from build123d import *

# Parameters (mm, degrees)
F1_DEPTH = 6
F2_R     = 3
F3_R     = 2.5
F4_DEPTH = 10
F5_R     = 2.5
F6_DEPTH = 10


with BuildPart() as f1:
    # F0 (on Right) → F1 (new body, symmetric)
    with BuildSketch(Plane.YZ):
        Polygon((0, 150), (-100, 0), (0, 0), align=None)
        Polygon((-10, 10), (-81.314829, 10), (-10, 116.972244), align=None, mode=Mode.SUBTRACT)
    extrude(amount=F1_DEPTH, both=True)

    # F2
    f2_edges = [f1.edges().sort_by_distance(p)[0] for p in [
        (0, -100, 0),
        (0, 0, 150),
        (0, -10, 116.972244),
        (0, -10, 10),
        (0, -81.314829, 10),
    ]]
    fillet(f2_edges, radius=F2_R)

    # F3 (on face) → F4 (cut, through all)
    with BuildSketch(Plane(origin=(0, 0, 0), x_dir=(-1, 0, 0), z_dir=(0, 1, 0))):
        with Locations((0, 90)):
            Circle(F3_R)
        with Locations((0, 25)):
            Circle(F3_R)
    extrude(amount=-F4_DEPTH, mode=Mode.SUBTRACT)

    # F5 (on face) → F6 (cut, through all)
    with BuildSketch(Plane(origin=(0, 0, 0), x_dir=(1, 0, 0), z_dir=(0, 0, -1))):
        with Locations((0, 25)):
            Circle(F5_R)
        with Locations((0, 65)):
            Circle(F5_R)
    extrude(amount=-F6_DEPTH, mode=Mode.SUBTRACT)


solid = f1.part
Here's how the part is built. I have some questions about the finished solid (model axes, mm). A direction names the side the tool comes from. Coordinates: 2 decimals unless noted, no trailing zeros. Loops run counter-clockwise (first coordinate to the right, second up) from the corner with the lowest first, then second, coordinate; pieces in that order, holes last. Notation, with made-up numbers: (4.25, 36) -> (43.25, 36) arc R22 cw to (43.25, 69) -> close; hole circle Ø9 at (17, 39.25). An arc over 180 degrees is marked (long way). Use one line per item in the form item = value. Start each with the question number.
(1) If we section it at D-D (y = -71): Please give me the cut outline in (x, z).
(2) Will these pins go through, and if not, where does the flat tip stop? pin 1 (3.5 mm diameter, centred on x = 1.5, z = 44.5, fed in from -Y); pin 2 (6 mm diameter, centred on x = 0.5, y = -60, fed in from +Z); pin 3 (3 mm diameter, centred on x = 0, y = -25, fed in from +Z).
(3) If we section it at C-C (x = 1): Please give me the cut outline in (y, z), then the cut area to 3 significant figures.
(4) Please list where these lines run through material, in increasing order: line 1 along Y through (x, z) = (0, 2.75); line 2 along Z through (x, y) = (0, -7.25) (3 decimals); line 3 along Y through (x, z) = (0, 6.75).
(5) We'd pull the mould along Z, two halves only. Please class faces 1 (the face through (-0.33, -27.48, 4.93)), 2 (the face through (0.084, -50.554, 74.17)), 3 (the face through (0.08, -10.9, 10.86)): pulls with the +Z half, pulls with the -Z half, needs draft (parallel to the pull), parting line crosses it, or undercut.
(6) If we section it at B-B (z = 71.5): Please give me the cut outline in (x, y), then the cut area to 3 significant figures.
(7) If we section it at A-A (y = -8.5): Please give me the cut outline in (x, z), then the cut area to 3 significant figures.
(8) On a 3-axis mill with a long thin cutter (end or side, diameter ignored), from which of +Z, -Z, +X, -X, +Y, -Y can I reach the whole of each face in a straight line? I mean faces 4 (the face through (0.33, -4.93, 27.48)), 5 (the face through (0.08, -47.29, 61.04)), 6 (the face through (-0.33, -67.48, 4.93)). Say none if no direction works.
Verdict:
q1.outline = (-6, 0) -> (6, 0) -> (6, 10) -> (-6, 10) -> close; (-6, 25.47) -> (6, 25.47) -> (6, 43.5) -> (-6, 43.5) -> close
q2.pin_1 = -71.5
q2.pin_2 = 64.5
q2.pin_3 = 114.75
q3.outline = (-96.89, 4.66) arc R3 ccw to (-94.39, 0) -> (-67.29, 0) -> (-67.29, 10) -> (-75.71, 10) arc R3 cw to (-78.21, 14.66) -> (-15.5, 108.73) arc R3 cw to (-10, 107.06) -> (-10, 92.29) -> (0, 92.29) -> (0, 140.09) arc R3 ccw to (-5.5, 141.76) -> close; (-62.71, 0) -> (-27.29, 0) -> (-27.29, 10) -> (-62.71, 10) -> close; (-22.71, 0) -> (0, 0) -> (0, 22.71) -> (-10, 22.71) -> (-10, 13) arc R3 cw to (-13, 10) -> (-22.71, 10) -> close; (-10, 27.29) -> (0, 27.29) -> (0, 87.71) -> (-10, 87.71) -> close
q3.area = 3,500 mm²
q4.line_1 = -97.38 to -67.5, -62.5 to -27.5, -22.5 to 0
q4.line_2 = 0 to 22.5, 27.5 to 87.5, 92.5 to 139.125
q4.line_3 = -95.5 to -67.5, -62.5 to -27.5, -22.5 to 0
q5.face_1 = needs draft
q5.face_2 = pulls with the +Z half
q5.face_3 = undercut
q6.outline = (-6, -52.33) -> (6, -52.33) -> (6, -40.31) -> (-6, -40.31) -> close; (-6, -10) -> (6, -10) -> (6, 0) -> (-6, 0) -> close
q6.area = 264 mm²
q7.outline = (-6, 0) -> (6, 0) -> (6, 137.25) -> (-6, 137.25) -> close; hole circle Ø5 at (0, 25); hole circle Ø5 at (0, 90)
q7.area = 1,610 mm²
q8.face_4 = +Y
q8.face_5 = +X, -X
q8.face_6 = -Z
